Here's how the part is built. I have some questions about the finished solid (model axes, mm). A direction names the side the tool comes from. Coordinates: 2 decimals unless noted, no trailing zeros. Write each loop counter-clockwise with the first axis right and the second up, starting at its lowest first coordinate (ties: lowest second). Pieces come first, ordered by that corner, then holes.
(1) Imagine slicing it at C-C, the plane z = -60.5. List the corners of the cut face in (x, y) for me.
(2) Thinking about a two-plate mould opening in Y: for faces 1 (the cylindrical face through (-0.644, 19.711, -25.804)), 2 (the flat face through (-1, 9, -30)), 3 (the flat face through (35, 83, -55)), which applies, released by +Y, released by -Y, zero draft, split by the parting line, or undercut?
(3) Which directions (+Z, -Z, +X, -X, +Y, -Y) give clear straight access to the entire face, cutting with the end or side of a thin tool? Please do faces 4 (the cylindrical face through (-26.227, 74.445, -21.021)), 5 (the flat face through (43, 77, -87)), 6 (the cylindrical face through (33.932, 10.605, 0.959)), 7 (the cylindrical face through (0.644, 65.587, -29.133)), 8 (the flat face through (27, 39, -12)).
(4) For pin 1 Ø0.9 at (x, z) = (-2.5, -35) entering from +Y; pin 2 Ø1 at (x, y) = (2, 89.5) entering from +Z; pin 3 Ø1.5 at (x, y) = (-4.5, 33) entering from +Z, each with a flat end and sliding along its axis, tell me the tip position at first contact or that it passes through.
(5) Please list where these lines run through material, in increasing order: probe 1 along X at (y, z) = (9, 2); probe 2 along Z at (x, y) = (-26, 6.75); probe 3 along X at (y, z) = (97, -87).
(6) Imagine slicing it at B-B, the plane z = -85. List the corners of the cut face in (x, y) for me.
```python
from build123d import *

# Parameters (mm, degrees)
CROQUIS1_W                   = 92
CROQUIS1_H                   = 60
SALIENTE_EXTRUIR1_DEPTH      = 18
CROQUIS2_R                   = 8
CORTAR_EXTRUIR1_DEPTH        = 15
SALIENTE_EXTRUIR2_DEPTH      = 92
REDONDEO1_R                  = 6
SALIENTE_EXTRUIR4_DEPTH      = 37
SALIENTE_EXTRUIR4_DEPTH_BACK = 18
CROQUIS4_R                   = 40
CROQUIS5_R                   = 20
CORTAR_EXTRUIR2_DEPTH        = 181.679273853
NERVIO1_START                = -7
NERVIO1_DEPTH                = 14
REDONDEO2_R                  = 42
REDONDEO3_R                  = 12


# Read off the part's stored shape, not the designer's step: Nervio1
with BuildPart() as part:
    # Croquis1 → Saliente-Extruir1 (new body)
    with BuildSketch(Plane(origin=(0, 0, 0), x_dir=(1, 0, 0), z_dir=(0, 1, 0))):
        Rectangle(CROQUIS1_W, CROQUIS1_H)
    extrude(amount=SALIENTE_EXTRUIR1_DEPTH)

    # Croquis2 → Cortar-Extruir1 (cut)
    with BuildSketch(Plane(origin=(0, 18, 0), x_dir=(1, 0, 0), z_dir=(0, 1, 0))):
        with Locations(Location((26, -2, 0), (0, 0, 270))):
            Circle(CROQUIS2_R)
        with Locations(Location((-26, -2, 0), (0, 0, 90))):
            Circle(CROQUIS2_R)
    extrude(amount=-CORTAR_EXTRUIR1_DEPTH, mode=Mode.SUBTRACT)

    # Croquis3 → Saliente-Extruir2 (add, through all)
    with BuildSketch(Plane(origin=(46, 0, 0), x_dir=(0, 0, -1), z_dir=(1, 0, 0))):
        with BuildLine():
            Line((18, 18), (24, 18))
            Line((24, 18), (24, 53))
            ThreePointArc((24, 53), (29.272077939, 65.727922061), (42, 71))
            Line((42, 71), (87, 71))
            Line((87, 71), (87, 83))
            Line((87, 83), (42, 83))
            ThreePointArc((42, 83), (20.786796564, 74.213203436), (12, 53))
            Line((12, 53), (12, 24))
            ThreePointArc((12, 24), (13.757359313, 19.757359313), (18, 18))
        make_face()
    extrude(amount=-SALIENTE_EXTRUIR2_DEPTH)

    # Redondeo1
    redondeo1_edges = [part.edges().sort_by_distance(p)[0] for p in [
        (0, 18, -24),
    ]]
    fillet(redondeo1_edges, radius=REDONDEO1_R - 0.0001)  # a hair under: the kernel refuses the full size

    # Croquis4 → Saliente-Extruir4 (add, two sides: drawn at the far end of the back side and taken through both)
    with BuildSketch(Plane(origin=(0, 83, 0), x_dir=(1, 0, 0), z_dir=(0, 1, 0)).offset(-SALIENTE_EXTRUIR4_DEPTH_BACK)):
        with Locations(Location((0, 87, 0), (0, 0, 270))):
            Circle(CROQUIS4_R)
    extrude(amount=SALIENTE_EXTRUIR4_DEPTH + SALIENTE_EXTRUIR4_DEPTH_BACK)

    # Croquis5 → Cortar-Extruir2 (cut, through all)
    with BuildSketch(Plane(origin=(0, 120, 0), x_dir=(1, 0, 0), z_dir=(0, 1, 0))):
        with Locations(Location((0, 87, 0), (0, 0, 270))):
            Circle(CROQUIS5_R)
    extrude(amount=-CORTAR_EXTRUIR2_DEPTH, mode=Mode.SUBTRACT)

    # Nervio1 outline → Nervio1 (add)
    with BuildSketch(Plane(origin=(0, 0, 0), x_dir=(0, 0, -1), z_dir=(1, 0, 0)).offset(NERVIO1_START)):
        with BuildLine():
            Line((42, 83), (48, 83))
            Line((48, 83), (48, 107))
            Line((48, 107), (6, 107))
            Line((6, 107), (-30, 18))
            Line((-30, 18), (18, 18))
            ThreePointArc((18, 18), (13.757359313, 19.757359313), (12, 24))
            Line((12, 24), (12, 53))
            ThreePointArc((12, 53), (20.786796564, 74.213203436), (42, 83))
        make_face()
    extrude(amount=NERVIO1_DEPTH)

    # Redondeo2
    redondeo2_edges = [part.edges().sort_by_distance(p)[0] for p in [
        (0, 107, -6),
    ]]
    fillet(redondeo2_edges, radius=REDONDEO2_R)

    # Redondeo3
    redondeo3_edges = [part.edges().sort_by_distance(p)[0] for p in [
        (-3.513581264, 107, -47.154614487),
    ]]
    fillet(redondeo3_edges, radius=REDONDEO3_R)


solid = part.part
```
Recorded:
1. outline: (-46, 71) - (-29.96, 71) - (-29.96, 65) - (29.96, 65) - (29.96, 71) - (46, 71) - (46, 83) - (29.96, 83) - (29.96, 120) - (-29.96, 120) - (-29.96, 83) - (-46, 83) - close
2. face 1: undercut
2. face 2: zero draft
2. face 3: released by +Y
3. face 4: +Z, -X, +Y
3. face 5: -Z, +X, +Y, -Y
3. face 6: +Y
3. face 7: +X, -X
3. face 8: +Z, +X, +Y
4. pin 1: stops at y = 107.01
4. pin 2: stops at z = 0.15
4. pin 3: stops at z = 24.24
5. probe 1: x = -46 to -34, -18 to 18, 34 to 46
5. probe 2: z = -30 to -6, 10 to 30
5. probe 3: x = -40 to -20, 20 to 40
6. outline: (-46, 71) - (-39.95, 71) - (-39.95, 65) - (-19.9, 65) - (-19.9, 120) - (-39.95, 120) - (-39.95, 83) - (-46, 83) - close; (19.9, 65) - (39.95, 65) - (39.95, 71) - (46, 71) - (46, 83) - (39.95, 83) - (39.95, 120) - (19.9, 120) - close
